```python
from build123d import *

# Parameters (mm, degrees)
SKETCH_1_W             = 234
SKETCH_1_H             = 130
EXTRUDE_1_DEPTH        = 90
SKETCH_2_W             = 78
SKETCH_2_H             = 118
CUT_EXTRUDE_1_DEPTH    = 283.411047943
SKETCH_3_R             = 13
CUT_EXTRUDE_2_DEPTH    = 283.411047943
PATTERN_LINEAR_1_COUNT = 3
PATTERN_LINEAR_1_PITCH = 80
SKETCH_4_R             = 13
CUT_EXTRUDE_3_DEPTH    = 283.411047943
PATTERN_LINEAR_2_COUNT = 3
PATTERN_LINEAR_2_PITCH = 80


with BuildPart() as part:
    # 草图1 → 凸台-拉伸1 (new body)
    with BuildSketch(Plane.XY):
        with Locations((117, 65)):
            Rectangle(SKETCH_1_W, SKETCH_1_H)
    extrude(amount=EXTRUDE_1_DEPTH)

    # 草图2 → 切除-拉伸1 (cut, through all)
    with BuildSketch(Plane.ZY):
        with Locations((51, 71)):
            Rectangle(SKETCH_2_W, SKETCH_2_H)
    extrude(amount=-CUT_EXTRUDE_1_DEPTH, mode=Mode.SUBTRACT)

    # 草图3 → 切除-拉伸2 (cut, through all)
    with BuildSketch(Plane(origin=(0, 0, 0), x_dir=(-1, 0, 0), z_dir=(0, 0, -1))):
        with Locations((-197, 80)):
            Circle(SKETCH_3_R)
    cut_extrude_2 = extrude(amount=-CUT_EXTRUDE_2_DEPTH, mode=Mode.SUBTRACT)

    # 阵列(线性)1: 切除-拉伸2 ×3
    with Locations(*[(-i * PATTERN_LINEAR_1_PITCH, 0, 0) for i in range(1, PATTERN_LINEAR_1_COUNT)]):
        add(cut_extrude_2, mode=Mode.SUBTRACT)

    # 草图4 → 切除-拉伸3 (cut, through all)
    with BuildSketch(Plane.XZ):
        with Locations(Location((37, 49, 0), (0, 0, 270))):
            Circle(SKETCH_4_R)
    cut_extrude_3 = extrude(amount=-CUT_EXTRUDE_3_DEPTH, mode=Mode.SUBTRACT)

    # 阵列(线性)2: 切除-拉伸3 ×3
    with Locations(*[(i * PATTERN_LINEAR_2_PITCH, 0, 0) for i in range(1, PATTERN_LINEAR_2_COUNT)]):
        add(cut_extrude_3, mode=Mode.SUBTRACT)


solid = part.part
```
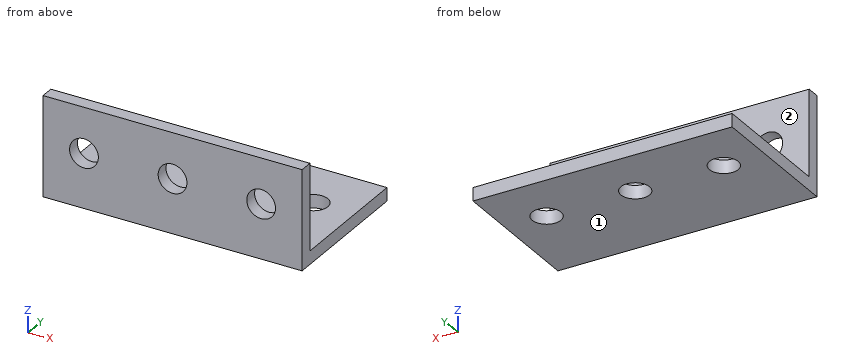
Verification items for the finished model (mm, model axes). Face numbers are marked on the shaded views. A direction names the side the tool comes from. Coordinates: 2 decimals unless noted, no trailing zeros. Write each loop counter-clockwise with the first axis right and the second up, starting at its lowest first coordinate (ties: lowest second). Pieces come first, ordered by that corner, then holes. Notation, with made-up numbers: M 39.5,89 L 59.5,89 A11 ccw 59.5,108 Z; hole C 71.25,12.25 d9. An arc over 180 degrees is marked long. One line per item, written item: value.
Item 1: Section check C-C, the plane x = 117. Record the boundary of the cut face in (y, z), plus the area to 3 significant figures.
Check sheet entries:
outline: M 0,0 L 67,0 L 67,12 L 12,12 L 12,36 L 0,36 Z; M 0,62 L 12,62 L 12,90 L 0,90 Z; M 93,0 L 130,0 L 130,12 L 93,12 Z
area: 1,870 mm^2
Item 2: Section check A-A, the plane y = 80. Record the boundary of the cut face in (x, z).
Check sheet entries:
outline: M 0,0 L 24,0 L 24,12 L 0,12 Z; M 50,0 L 104,0 L 104,12 L 50,12 Z; M 130,0 L 184,0 L 184,12 L 130,12 Z; M 210,0 L 234,0 L 234,12 L 210,12 Z
Item 3: Access from +Z, -Z, +X, -X, +Y, -Y to the whole of each face (thin tool, end or side, straight path). Record for the marked faces 1 and 2.
Check sheet entries:
face 1: -Z, +X, -X, +Y, -Y
face 2: +Z, +X, -X, +Y
Item 4: Gauge pin test, flat ends, axial feed: pin 1 Ø6 at (x, y) = (72, 50) entering from -Z; pin 2 Ø10 at (x, y) = (100, 96) entering from +Z; pin 3 Ø4 at (x, z) = (184, 60.5) entering from +Y. Record the tip position at first contact, or that the pin passes through.
Check sheet entries:
pin 1: stops at z = 0
pin 2: stops at z = 12
pin 3: stops at y = 12
Item 5: Scan lines: line 1 along X through (y, z) = (4.5, 49); line 2 along Y through (x, z) = (117, 6.5); line 3 along Z through (x, y) = (60, 48). Record each from-to range of solid material in increasing order.
Check sheet entries:
line 1: x = 0 to 24, 50 to 104, 130 to 184, 210 to 234
line 2: y = 0 to 67, 93 to 130
line 3: z = 0 to 12
Item 6: Section check D-D, the plane y = 8.5. Record the boundary of the cut face in (x, z).
Check sheet entries:
outline: M 0,0 L 234,0 L 234,90 L 0,90 Z; hole C 37,49 d26; hole C 117,49 d26; hole C 197,49 d26
